from build123d import *

# Parameters (mm, degrees)
SKETCH1_R           = 1.6
BOSS_EXTRUDE1_DEPTH = 6.5
FILLET1_R           = 10
SKETCH2_W           = 17.85
SKETCH2_H           = 4.708375864
CUT_EXTRUDE1_DEPTH  = 4.5


with BuildPart() as part:
    # Sketch1 → Boss-Extrude1 (new body)
    with BuildSketch(Plane(origin=(0, 0, 0), x_dir=(1, 0, 0), z_dir=(0, 1, 0))):
        with BuildLine():
            Line((9.827855615, 2), (-9.827855615, 2))
            ThreePointArc((-9.827855615, 2), (-16.75, 0), (-9.827855615, -2))
            Line((-9.827855615, -2), (9.827855615, -2))
            ThreePointArc((9.827855615, -2), (16.75, 0), (9.827855615, 2))
        make_face()
        with Locations(Location((-13, 0, 0), (0, 0, 90))):
            Circle(SKETCH1_R, mode=Mode.SUBTRACT)
        with Locations(Location((13, 0, 0), (0, 0, 90))):
            Circle(SKETCH1_R, mode=Mode.SUBTRACT)
    extrude(amount=BOSS_EXTRUDE1_DEPTH)

    # Fillet1
    fillet1_edges = [part.edges().sort_by_distance(p)[0] for p in [
        (-9.827855615, 3.25, -2),
        (9.827855615, 3.25, -2),
        (9.827855615, 3.25, 2),
        (-9.827855615, 3.25, 2),
    ]]
    fillet(fillet1_edges, radius=FILLET1_R)

    # Sketch2 → Cut-Extrude1 (cut)
    with BuildSketch(Plane(origin=(0, 0, 0), x_dir=(-1, 0, 0), z_dir=(0, -1, 0))):
        Rectangle(SKETCH2_W, SKETCH2_H)
    extrude(amount=-CUT_EXTRUDE1_DEPTH, mode=Mode.SUBTRACT)


solid = part.part
Model file for the job. Use its own axes, mm. A direction names the side the tool comes from. Give positions to 0.01 mm unless a question says otherwise; leave off trailing zeros. Order: outer loops, then holes, each group sorted by start corner. A loop starts at its lowest first (then second) coordinate and runs counter-clockwise, first axis right, second up. Notation, with made-up numbers: M 59.5,-23.75 L 108.5,-23.75 A31 cw 108.5,6.25 Z; hole C -17.5,8.5 d3. An arc over 180 degrees is marked long. Write item = value, one per line.
Q1. Cut at D-D, the plane y = 5.5. List the corners of the cut face in (x, z).
Derived:
outline = M -11.17,-3.27 A10 cw -6.29,-2 L 6.29,-2 A10 cw 11.17,-3.27 A3.75 ccw long 11.17,3.27 A10 cw 6.29,2 L -6.29,2 A10 cw -11.17,3.27 A3.75 ccw long Z; hole C -13,0 d3.2; hole C 13,0 d3.2
Q2. Cut at C-C, the plane z = 0. List the corners of the cut face in (x, y) (3 decimals).
Derived:
outline = M -16.75,0 L -14.6,0 L -14.6,6.5 L -16.75,6.5 Z; M -11.4,0 L -8.925,0 L -8.925,4.5 L 8.925,4.5 L 8.925,0 L 11.4,0 L 11.4,6.5 L -11.4,6.5 Z; M 14.6,0 L 16.75,0 L 16.75,6.5 L 14.6,6.5 Z
Q3. Flat gauge pins, fed straight in: pin 1 (2 mm diameter, centred on x = -2, y = 4, fed in from -Z); pin 2 (1.5 mm diameter, centred on x = 11.5, y = 3.5, fed in from -Z); pin 3 (1.6 mm diameter, centred on x = 2.5, y = 6, fed in from +Z); pin 4 (3 mm diameter, centred on x = 13, z = 0, fed in from -Y). Where does each tip first touch, or does it go through?
Derived:
pin_1 = -2
pin_2 = -3.67
pin_3 = 2
pin_4 = through
Q4. Tool access for faces 4 (the flat face through (-13, 0, 2)), 5 (the flat face through (-8.925, 2, 0)), 6 (the cylindrical face through (-14.586, 3.204, 0.208)), 7 (the cylindrical face through (-9.388, 4.018, 2.493)), 8 (the flat face through (0, 5, -2)): list every direction of +Z, -Z, +X, -X, +Y, -Y with a clear straight run to the whole face (end or side of a thin tool).
Derived:
face_4 = +Z, -Z, +X, -X, -Y
face_5 = +Z, -Z, -Y
face_6 = +Y, -Y
face_7 = +Z, +Y, -Y
face_8 = -Z, +Y, -Y
Q5. Drill centre lines: line 1 (X direction, y = 3.75, z = 0) (3 decimals); line 2 (X direction, y = 5, z = 0); line 3 (Z direction, x = -13, y = 2). Where is each one in solid material? Low to high. Write a range as [from, to].
Derived:
line_1 = [-16.75, -14.6], [-11.4, -8.925], [8.925, 11.4], [14.6, 16.75]
line_2 = [-16.75, -14.6], [-11.4, 11.4], [14.6, 16.75]
line_3 = [-3.75, -1.6], [1.6, 3.75]
Q6. Cut at B-B, the plane x = 13. List the corners of the cut face in (y, z), then the cut area to 4 significant figures.
Derived:
outline = M 0,-3.75 L 6.5,-3.75 L 6.5,-1.6 L 0,-1.6 Z; M 0,1.6 L 6.5,1.6 L 6.5,3.75 L 0,3.75 Z
area = 27.95 mm2
Q7. Two-plate mould, pull along X, no slides. Class faces 1 (the flat face through (13, 0, 2)), 2 (the cylindrical face through (-9.32, 4.02, -2.47)), 3 (the flat face through (8.925, 2, 0)): pulls with the +X half, pulls with the -X half, needs draft (parallel to the pull), parting line crosses it, or undercut.
Derived:
face_1 = needs draft
face_2 = undercut
face_3 = undercut
Q8. Cut at A-A, the plane y = 0.5. List the corners of the cut face in (x, z) (3 decimals).
Derived:
outline = M -11.169,-3.273 A10 cw -8.925,-2.354 L -8.925,2.354 A10 cw -11.169,3.273 A3.75 ccw long Z; M 8.925,-2.354 A10 cw 11.169,-3.273 A3.75 ccw long 11.169,3.273 A10 cw 8.925,2.354 Z; hole C -13,0 d3.2; hole C 13,0 d3.2
